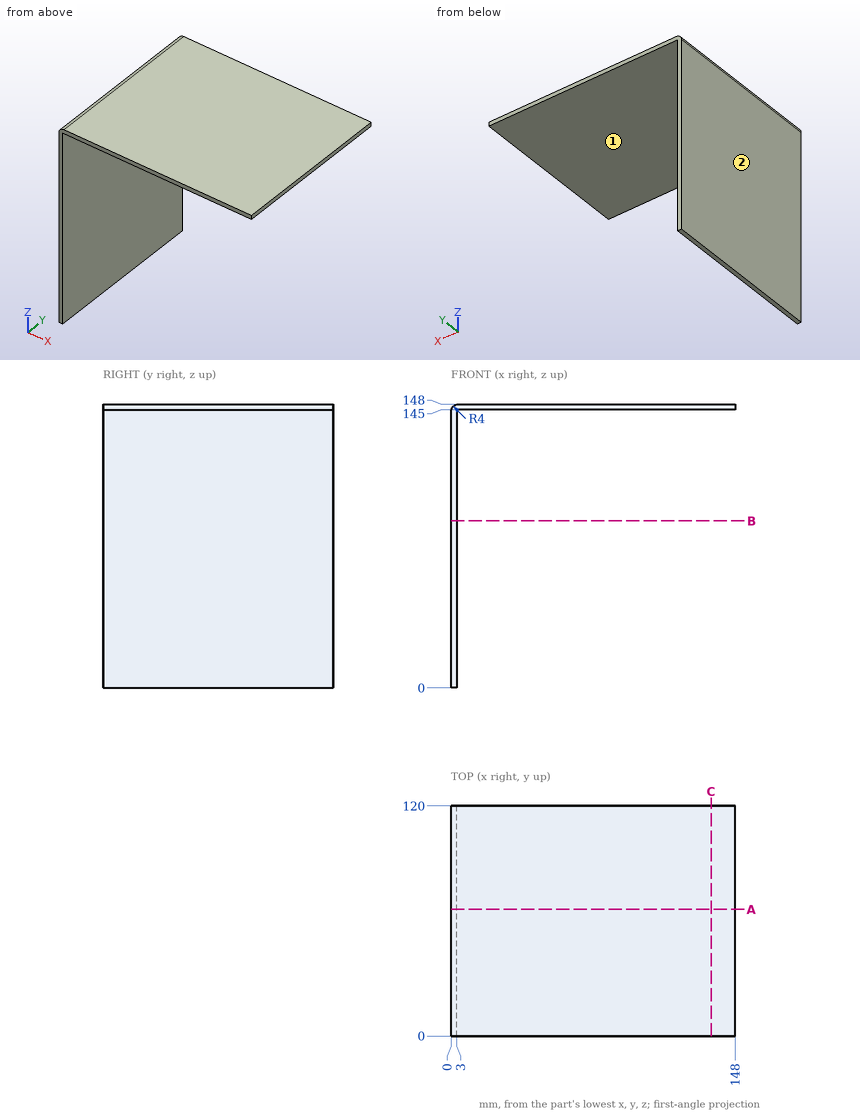
Verification items for this drawing (mm, ordinates from the low corner). A direction names the side the tool comes from. Coordinates: 2 decimals unless noted, no trailing zeros. Write each loop counter-clockwise with the first axis right and the second up, starting at its lowest first coordinate (ties: lowest second). Pieces come first, ordered by that corner, then holes. Notation, with made-up numbers: (31, 84.25) -> (35, 84.25) arc R8 ccw to (35, 94.25) -> close; hole circle Ø11 at (9, 75). An arc over 180 degrees is marked (long way). One line per item, written item: value. Start each with the question number.
Q1. Cross-section at B-B on z = 87. Enter the section's corners in (x, y), and give its area (3 significant figures).
Q2. Access from +Z, -Z, +X, -X, +Y, -Y to the whole of each face (thin tool, end or side, straight path). Record for the marked faces 1 and 2.
Q3. Cross-section at A-A on y = 66. Enter the section's corners in (x, z).
Q4. Go/stop test with flat-tipped pins: P1, Ø4, axis at y = 79, z = 23, coming from the +X side; P2, Ø5, axis at x = 41.5, y = 65.5, coming from the -Z side. Record where each tip stops, or that it passes through.
Q5. Thickness scan on L1, parallel to Z at x = 12, y = 13.5; L2, parallel to X at y = 114, z = 99.5. Record the ranges inside material, lowest first. Write a range as from..to.
Q6. Cross-section at C-C on x = 135.5. Enter the section's corners in (y, z).
Checked values:
1. outline: (0, 0) -> (3, 0) -> (3, 120) -> (0, 120) -> close
1. area: 360 mm²
2. face 1: -Z, +X, +Y, -Y
2. face 2: +Z, -Z, -X, +Y, -Y
3. outline: (0, 0) -> (3, 0) -> (3, 145) -> (148, 145) -> (148, 148) -> (4, 148) arc R4 ccw to (0, 144) -> close
4. P1: stops at x = 3
4. P2: stops at z = 145
5. L1: z = 145..148
5. L2: x = 0..3
6. outline: (0, 145) -> (120, 145) -> (120, 148) -> (0, 148) -> close
